```python
from build123d import *

# Parameters (mm, degrees)
SKETCH1_W                 = 48.5775
SKETCH1_H                 = 58.7375
BOSS_EXTRUDE1_DEPTH       = 34.13125
SKETCH2_W                 = 21.9075
SKETCH2_H                 = 53.975
CUT_EXTRUDE1_DEPTH        = 2.38125
SKETCH4_W                 = 14.2875
SKETCH4_H                 = 53.975
CUT_EXTRUDE2_DEPTH        = 29.36875
SKETCH5_W                 = 7.62
SKETCH5_H                 = 53.975
CUT_EXTRUDE3_DEPTH        = 13.0175
F_4_40_TAPPED_HOLE1_D     = 2.2606
F_4_40_TAPPED_HOLE1_DEPTH = 16.35125
F_4_40_TAPPED_HOLE1_TIP   = 0.679152758
FILLET3_R                 = 2.032
FILLET4_R                 = 2.032


with BuildPart() as part:
    # Sketch1 → Boss-Extrude1 (new body)
    with BuildSketch(Plane.XY):
        with Locations((0, -29.36875)):
            Rectangle(SKETCH1_W, SKETCH1_H)
    extrude(amount=BOSS_EXTRUDE1_DEPTH)

    # Sketch2 → Cut-Extrude1 (cut)
    with BuildSketch(Plane.XY.offset(34.13125)):
        with Locations((10.95375, -29.36875)):
            Rectangle(SKETCH2_W, SKETCH2_H)
        with Locations((-10.95375, -29.36875)):
            Rectangle(SKETCH2_W, SKETCH2_H)
    extrude(amount=-CUT_EXTRUDE1_DEPTH, mode=Mode.SUBTRACT)

    # Sketch4 → Cut-Extrude2 (cut)
    with BuildSketch(Plane.XY.offset(31.75)):
        with Locations((7.14375, -29.36875)):
            Rectangle(SKETCH4_W, SKETCH4_H)
        with Locations((-7.14375, -29.36875)):
            Rectangle(SKETCH4_W, SKETCH4_H)
    extrude(amount=-CUT_EXTRUDE2_DEPTH, mode=Mode.SUBTRACT)

    # Sketch5 → Cut-Extrude3 (cut)
    with BuildSketch(Plane.XY.offset(31.75)):
        with Locations((-18.0975, -29.36875)):
            Rectangle(SKETCH5_W, SKETCH5_H)
        with Locations((18.0975, -29.36875)):
            Rectangle(SKETCH5_W, SKETCH5_H)
    extrude(amount=-CUT_EXTRUDE3_DEPTH, mode=Mode.SUBTRACT)

    # #4-40 Tapped Hole1
    with Locations(Plane.XY.offset(18.7325)):
        with Locations((-14.8082, -16.2521392), (-14.8082, -42.4853608), (14.8082, -42.4853608), (14.8082, -16.2521392)):
            Hole(F_4_40_TAPPED_HOLE1_D / 2, depth=F_4_40_TAPPED_HOLE1_DEPTH)
            with Locations((0, 0, -(F_4_40_TAPPED_HOLE1_DEPTH + F_4_40_TAPPED_HOLE1_TIP / 2))):  # 118° drill point
                Cone(0, F_4_40_TAPPED_HOLE1_D / 2, F_4_40_TAPPED_HOLE1_TIP, mode=Mode.SUBTRACT)

    # Fillet3
    fillet3_edges = [part.edges().sort_by_distance(p)[0] for p in [
        (-24.28875, -29.36875, 34.13125),
    ]]
    fillet(fillet3_edges, radius=FILLET3_R)

    # Fillet4
    fillet4_edges = [part.edges().sort_by_distance(p)[0] for p in [
        (-24.28875, -58.7375, 16.049625),
        (-23.693590979, -58.7375, 33.536090979),
        (-24.28875, 0, 16.049625),
        (-23.693590979, 0, 33.536090979),
        (1.016, 0, 34.13125),
        (24.28875, -29.36875, 34.13125),
        (0, 0, 0),
        (-24.28875, -29.36875, 0),
        (0, -58.7375, 0),
        (24.28875, -29.36875, 0),
        (1.016, -58.7375, 34.13125),
        (24.28875, 0, 17.065625),
        (24.28875, -58.7375, 17.065625),
    ]]
    fillet(fillet4_edges, radius=FILLET4_R)


solid = part.part
```
Geometry check sheet. Reference: the model listing, model coordinates, mm. A direction names the side the tool comes from. Coordinates: 2 decimals unless noted, no trailing zeros. Order: outer loops, then holes, each group sorted by start corner. A loop starts at its lowest first (then second) coordinate and runs counter-clockwise, first axis right, second up.
Item 1: Mould release check, pull along Y, two halves, no side actions. Record for faces 1 (the flat face through (0, -58.738, 17)), 2 (the flat face through (-18, -29, 18.732)), 3 (the cylindrical face through (0.31, -0.61, 33.55)), 4 (the flat face through (0, -29, 2.381)): released by +Y, released by -Y, zero draft, split by the parting line, or undercut.
Item 2: Section check A-A (z = 17.5). Enter the section's corners in (x, y).
Item 3: Depth check by flat-ended pin: pin 1 (23 mm diameter, centred on x = 2.5, y = -42, fed in from +Z); pin 2 (2 mm diameter, centred on x = -14.5, y = -43.5, fed in from +Z); pin 3 (2 mm diameter, centred on x = -14.81, y = -42.49, fed in from +Z). Enter the tip coordinate at first touch or a pass-through.
Item 4: Tool access check on faces 5 (the cylindrical face through (-23.709, -58.126, 17.276)), 6 (the flat face through (-14.288, -50, 11)). Record the directions out of +Z, -Z, +X, -X, +Y, -Y that give a thin tool (end or side, any length) a straight path to the whole face; none if there is none.
Item 5: Section check D-D (z = 24). Enter the section's corners in (x, y), plus the area to 3 significant figures.
Item 6: Section check C-C (x = 4). Enter the section's corners in (y, z).
Item 7: Section check B-B (y = -31). Enter the section's corners in (x, z).
Item 8: Scan lines: line 1 along X through (y, z) = (-49, 12.5); line 2 along Y through (x, z) = (-8.5, 7); line 3 along X through (y, z) = (-4, 22.5). Record each from-to range of solid material in increasing order.
Check sheet entries:
1. face 1: released by -Y
1. face 2: undercut
1. face 3: released by +Y
1. face 4: undercut
2. outline: (-24.29, -56.71) arc R2.03 ccw to (-22.26, -58.74) - (22.26, -58.74) arc R2.03 ccw to (24.29, -56.71) - (24.29, -2.03) arc R2.03 ccw to (22.26, 0) - (-22.26, 0) arc R2.03 ccw to (-24.29, -2.03) - close; hole (-14.29, -56.36) - (14.29, -56.36) - (14.29, -43.49) arc R1.13 ccw (long way) to (14.29, -41.48) - (14.29, -17.26) arc R1.13 ccw (long way) to (14.29, -15.25) - (14.29, -2.38) - (-14.29, -2.38) - (-14.29, -15.25) arc R1.13 ccw (long way) to (-14.29, -17.26) - (-14.29, -41.48) arc R1.13 ccw (long way) to (-14.29, -43.49) - close
3. pin 1: stops at z = 2.38
3. pin 2: stops at z = 18.73
3. pin 3: stops at z = 2.31
4. face 5: +Z, -Z, -X, -Y
4. face 6: +Z
5. outline: (-24.29, -56.71) arc R2.03 ccw to (-22.26, -58.74) - (22.26, -58.74) arc R2.03 ccw to (24.29, -56.71) - (24.29, -2.03) arc R2.03 ccw to (22.26, 0) - (-22.26, 0) arc R2.03 ccw to (-24.29, -2.03) - close; hole (-21.91, -56.36) - (21.91, -56.36) - (21.91, -2.38) - (-21.91, -2.38) - close
5. area: 485 mm2
6. outline: (-58.74, 2.03) arc R2.03 ccw to (-56.71, 0) - (-2.03, 0) arc R2.03 ccw to (0, 2.03) - (0, 32.1) arc R2.03 ccw to (-2.03, 34.13) - (-2.38, 34.13) - (-2.38, 2.38) - (-56.36, 2.38) - (-56.36, 34.13) - (-56.71, 34.13) arc R2.03 ccw to (-58.74, 32.1) - close
7. outline: (-24.29, 2.03) arc R2.03 ccw to (-22.26, 0) - (22.26, 0) arc R2.03 ccw to (24.29, 2.03) - (24.29, 32.1) arc R2.03 ccw to (22.26, 34.13) - (21.91, 34.13) - (21.91, 18.73) - (14.29, 18.73) - (14.29, 2.38) - (-14.29, 2.38) - (-14.29, 18.73) - (-21.91, 18.73) - (-21.91, 34.13) - (-22.26, 34.13) arc R2.03 ccw to (-24.29, 32.1) - close
8. line 1: x = -24.29 to -14.29, 14.29 to 24.29
8. line 2: y = -58.74 to -56.36, -2.38 to 0
8. line 3: x = -24.29 to -21.91, 21.91 to 24.29
